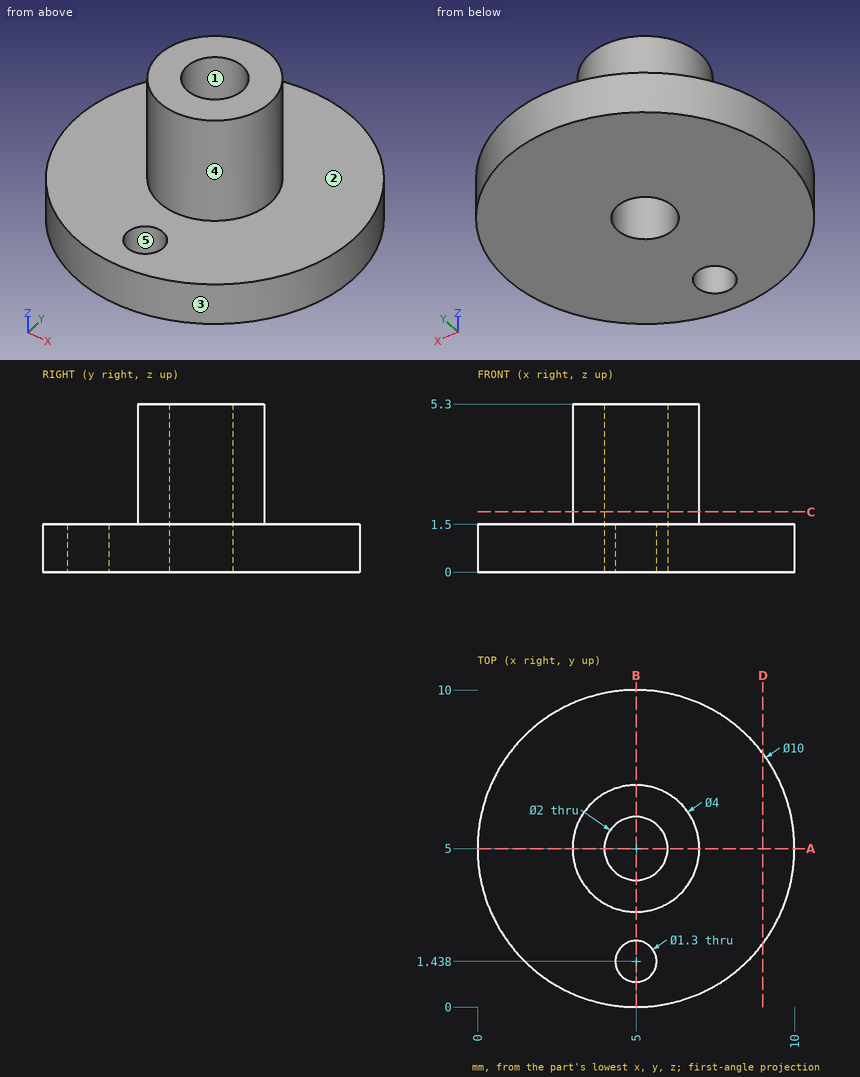
Verification items for this drawing (mm, ordinates from the low corner). A direction names the side the tool comes from. Give positions to 0.01 mm unless a question says otherwise; leave off trailing zeros. Loops run counter-clockwise (first coordinate to the right, second up) from the corner with the lowest first, then second, coordinate; pieces in that order, holes last. Notation, with made-up numbers: M 71.5,61.5 L 79.5,61.5 A20 ccw 79.5,98.5 Z; hole C 74,-21.75 d1. An arc over 180 degrees is marked long. Return JSON: item names as keys, results as strings. Group by question number.
1. Cross-section at D-D on x = 9. Record the boundary of the cut face in (y, z).
2. Mould release check, pull along Y, two halves, no side actions. Record for the marked faces 1, 2 and 3: released by +Y, released by -Y, zero draft, split by the parting line, or undercut.
3. Cross-section at B-B on x = 5. Record the boundary of the cut face in (y, z).
4. Tool access check on the marked faces 4 and 5. Record the directions out of +Z, -Z, +X, -X, +Y, -Y that give a thin tool (end or side, any length) a straight path to the whole face; none if there is none.
5. Thickness scan on L1, parallel to Y at x = 5, z = 0.5; L2, parallel to Y at x = 4.5, z = 1.15 (1 decimal); L3, parallel to Y at x = 5, z = 2.05. Record the ranges inside material, lowest first.
6. Cross-section at A-A on y = 5. Record the boundary of the cut face in (x, z), plus the area to 3 significant figures.
7. Cross-section at C-C on z = 1.9. Record the boundary of the cut face in (x, y).
8. Go/stop test with flat-tipped pins: pin 1 (2 mm diameter, centred on y = 6.5, z = 1.5, fed in from -X) (1 decimal); pin 2 (1 mm diameter, centred on x = 5, y = 1.44, fed in from +Z); pin 3 (1 mm diameter, centred on x = 3, z = 4, fed in from +Y); pin 4 (1.5 mm diameter, centred on x = 3.5, z = 3.5, fed in from -Y). Record where each tip stops, or that it passes through.
Return value:
{
 "1": {"outline": "M 2,0 L 8,0 L 8,1.5 L 2,1.5 Z"},
 "2": {"face 1": "undercut", "face 2": "zero draft", "face 3": "split by the parting line"},
 "3": {"outline": "M 0,0 L 0.79,0 L 0.79,1.5 L 0,1.5 Z; M 2.09,0 L 4,0 L 4,5.3 L 3,5.3 L 3,1.5 L 2.09,1.5 Z; M 6,0 L 10,0 L 10,1.5 L 7,1.5 L 7,5.3 L 6,5.3 Z"},
 "4": {"face 4": "+Z", "face 5": "+Z, -Z"},
 "5": {"L1": "0 to 0.79, 2.09 to 4, 6 to 10", "L2": "0 to 1, 1.9 to 4.1, 5.9 to 10", "L3": "3 to 4, 6 to 7"},
 "6": {"outline": "M 0,0 L 4,0 L 4,5.3 L 3,5.3 L 3,1.5 L 0,1.5 Z; M 6,0 L 10,0 L 10,1.5 L 7,1.5 L 7,5.3 L 6,5.3 Z", "area": "19.6 mm^2"},
 "7": {"outline": "C 5,5 d4; hole C 5,5 d2"},
 "8": {"pin 1": "x = 0", "pin 2": "through", "pin 3": "y = 6.32", "pin 4": "y = 3.15"}
}
